```python
from build123d import *

# Parameters (mm, degrees)
SKETCH1_W            = 3.556
SKETCH1_H            = 2.794
SKETCH1_W_2          = 1.3716
SKETCH1_H_2          = 0.635
BOSS_EXTRUDE1_DEPTH  = 34.29
SKETCH2_R            = 9.525
BOSS_EXTRUDE2_DEPTH  = 8.255
SKETCH3_R            = 4.0005
BOSS_EXTRUDE3_DEPTH  = 13.081
SKETCH4_W            = 25.4
SKETCH4_H            = 16.9037
BOSS_EXTRUDE4_DEPTH  = 21.6662
SKETCH5_R            = 4.0005
BOSS_EXTRUDE5_DEPTH  = 13.081
SKETCH6_R            = 9.525
BOSS_EXTRUDE6_DEPTH  = 3.81
SKETCH7_W            = 19.177
SKETCH7_H            = 19.177
BOSS_EXTRUDE7_DEPTH  = 5.08
SKETCH8_R            = 3.175
BOSS_EXTRUDE8_DEPTH  = 15.494
SKETCH9_W            = 6.35
SKETCH9_H            = 6.35
BOSS_EXTRUDE9_DEPTH  = 6.35
SKETCH10_R           = 3.175
BOSS_EXTRUDE10_DEPTH = 3.175
BOSS_EXTRUDE11_DEPTH = 15.24
SKETCH12_R           = 3.175
BOSS_EXTRUDE12_DEPTH = 6.985
SKETCH13_W           = 15.9004
SKETCH13_H           = 15.875
BOSS_EXTRUDE13_DEPTH = 2.54
BOSS_EXTRUDE15_DEPTH = 2.54
CUT_EXTRUDE1_DEPTH   = 15
CUT_EXTRUDE2_DEPTH   = 15
FILLET1_R            = 1.27
SKETCH22_R           = 2.54
SKETCH22_R_2         = 0.127
CUT_EXTRUDE3_DEPTH   = 3.81
SKETCH22_3_R         = 0.127
CUT_EXTRUDE4_DEPTH   = 12.7
CUT_EXTRUDE7_DEPTH   = 5.08


with BuildPart() as part:
    # Sketch1 → Boss-Extrude1 (new body)
    with BuildSketch(Plane(origin=(0, 0, 0), x_dir=(1, 0, 0), z_dir=(0, 1, 0))):
        with Locations((1.778, -1.397)):
            Rectangle(SKETCH1_W, SKETCH1_H)
        with Locations((1.778, -1.397)):
            Rectangle(SKETCH1_W_2, SKETCH1_H_2, mode=Mode.SUBTRACT)
    extrude(amount=BOSS_EXTRUDE1_DEPTH)

    # Sketch2 → Boss-Extrude2 (add)
    with BuildSketch(Plane(origin=(0, 34.29, 0), x_dir=(1, 0, 0), z_dir=(0, 1, 0))):
        with Locations((1.778, -1.397)):
            Circle(SKETCH2_R)
    extrude(amount=BOSS_EXTRUDE2_DEPTH)

    # Sketch3 → Boss-Extrude3 (add)
    with BuildSketch(Plane(origin=(0, 42.545, 0), x_dir=(1, 0, 0), z_dir=(0, 1, 0))):
        with Locations((1.778, -1.397)):
            Circle(SKETCH3_R)
    extrude(amount=BOSS_EXTRUDE3_DEPTH)

    # Sketch4 → Boss-Extrude4 (add)
    with BuildSketch(Plane(origin=(0, 55.626, 0), x_dir=(1, 0, 0), z_dir=(0, 1, 0))):
        with Locations((1.778, -1.397)):
            Rectangle(SKETCH4_W, SKETCH4_H)
    extrude(amount=BOSS_EXTRUDE4_DEPTH)

    # Sketch5 → Boss-Extrude5 (add)
    with BuildSketch(Plane(origin=(0, 77.2922, 0), x_dir=(1, 0, 0), z_dir=(0, 1, 0))):
        with Locations((1.778, -1.397)):
            Circle(SKETCH5_R)
    extrude(amount=BOSS_EXTRUDE5_DEPTH)

    # Sketch6 → Boss-Extrude6 (add)
    with BuildSketch(Plane(origin=(0, 90.3732, 0), x_dir=(1, 0, 0), z_dir=(0, 1, 0))):
        with Locations((1.778, -1.397)):
            Circle(SKETCH6_R)
    extrude(amount=BOSS_EXTRUDE6_DEPTH)

    # Sketch7 → Boss-Extrude7 (add)
    with BuildSketch(Plane(origin=(0, 94.1832, 0), x_dir=(1, 0, 0), z_dir=(0, 1, 0))):
        with Locations((1.778, -1.397)):
            Rectangle(SKETCH7_W, SKETCH7_H)
    extrude(amount=BOSS_EXTRUDE7_DEPTH)

    # Sketch8 → Boss-Extrude8 (add)
    with BuildSketch(Plane(origin=(0, 99.2632, 0), x_dir=(1, 0, 0), z_dir=(0, 1, 0))):
        with Locations((1.778, 3.39725)):
            Circle(SKETCH8_R)
    extrude(amount=BOSS_EXTRUDE8_DEPTH)

    # Sketch9 → Boss-Extrude9 (add)
    with BuildSketch(Plane(origin=(0, 114.7572, 0), x_dir=(1, 0, 0), z_dir=(0, 1, 0))):
        with Locations((1.778, 3.39725)):
            Rectangle(SKETCH9_W, SKETCH9_H)
    extrude(amount=BOSS_EXTRUDE9_DEPTH)

    # Sketch10 → Boss-Extrude10 (add)
    with BuildSketch(Plane(origin=(0, 0, -6.57225), x_dir=(-1, 0, 0), z_dir=(0, 0, -1))):
        with Locations((-1.778, 117.9322)):
            Circle(SKETCH10_R)
    extrude(amount=BOSS_EXTRUDE10_DEPTH)

    # Sketch11 → Boss-Extrude11 (add)
    with BuildSketch(Plane(origin=(0, 0, -9.74725), x_dir=(-1, 0, 0), z_dir=(0, 0, -1))):
        Polygon((0.49502801, 113.9952), (2.76805602, 117.9322), (0.49502801, 121.8692), (-4.05102801, 121.8692), (-6.32405602, 117.9322), (-4.05102801, 113.9952), align=None)
    extrude(amount=BOSS_EXTRUDE11_DEPTH)

    # Sketch12 → Boss-Extrude12 (add)
    with BuildSketch(Plane(origin=(0, 0, -24.98725), x_dir=(-1, 0, 0), z_dir=(0, 0, -1))):
        with Locations((-1.778, 117.9322)):
            Circle(SKETCH12_R)
    extrude(amount=BOSS_EXTRUDE12_DEPTH)

    # Sketch13 → Boss-Extrude13 (add)
    with BuildSketch(Plane(origin=(0, 0, -7.05485), x_dir=(-1, 0, 0), z_dir=(0, 0, -1))):
        with Locations((-5.2578, 66.8147)):
            Rectangle(SKETCH13_W, SKETCH13_H)
    extrude(amount=BOSS_EXTRUDE13_DEPTH)

    # Sketch16 → Revolve1 (revolve)
    with BuildSketch(Plane(origin=(5.2578, 0, 0), x_dir=(0, 0, -1), z_dir=(1, 0, 0))):
        with BuildLine():
            Line((9.59485, 66.8147), (9.59485, 71.8947))
            Line((9.59485, 71.8947), (16.19885, 71.8947))
            Line((16.19885, 71.8947), (17.97685, 73.1647))
            Line((17.97685, 73.1647), (25.08885, 73.1647))
            Line((25.08885, 73.1647), (25.08885, 73.6727))
            Line((25.08885, 73.6727), (31.43885, 73.6727))
            ThreePointArc((31.43885, 73.6727), (33.469498821, 71.155053903), (34.48685, 68.0847))
            Line((34.48685, 68.0847), (34.74085, 68.0847))
            Line((34.74085, 68.0847), (34.74085, 66.8147))
            Line((34.74085, 66.8147), (9.59485, 66.8147))
        make_face()
    revolve(axis=Axis((5.2578, 66.8147, -9.59485), (0, 0, -1)))

    # Sketch17 → Boss-Extrude15 (add, symmetric)
    with BuildSketch(Plane(origin=(0, 107.0102, 0), x_dir=(1, 0, 0), z_dir=(0, 1, 0))):
        Polygon((6.470702988, 3.39725), (4.124351494, 7.46125), (-0.568351494, 7.46125), (-2.914702988, 3.39725), (-0.568351494, -0.66675), (4.124351494, -0.66675), align=None)
    extrude(amount=BOSS_EXTRUDE15_DEPTH, both=True)

    # Sketch20 → Cut-Extrude1 (cut)
    with BuildSketch(Plane.ZY):
        Polygon((0, 0), (0.762, 0), (0, 1.27), align=None)
        Polygon((2.794, 0), (2.794, 1.27), (2.032, 0), align=None)
    extrude(amount=-CUT_EXTRUDE1_DEPTH, mode=Mode.SUBTRACT)

    # Sketch21 → Cut-Extrude2 (cut)
    with BuildSketch(Plane(origin=(0, 0, 0), x_dir=(-1, 0, 0), z_dir=(0, 0, -1))):
        Polygon((-3.556, 1.27), (-3.556, 0), (-2.794, 0), align=None)
        Polygon((0, 1.27), (-0.762, 0), (0, 0), align=None)
    extrude(amount=-CUT_EXTRUDE2_DEPTH, mode=Mode.SUBTRACT)

    # Fillet1
    fillet1_edges = [part.edges().sort_by_distance(p)[0] for p in [
        (1.778, 34.29, 0),
        (0, 34.29, 1.397),
        (1.778, 34.29, 2.794),
        (3.556, 34.29, 1.397),
    ]]
    fillet(fillet1_edges, radius=FILLET1_R)

    # Sketch22 → Cut-Extrude3 (cut)
    with BuildSketch(Plane(origin=(0, 0, -31.97225), x_dir=(-1, 0, 0), z_dir=(0, 0, -1))):
        with Locations((-1.778, 117.9322)):
            Circle(SKETCH22_R)
        with Locations((-1.778, 117.9322)):
            Circle(SKETCH22_R_2, mode=Mode.SUBTRACT)
    extrude(amount=-CUT_EXTRUDE3_DEPTH, mode=Mode.SUBTRACT)

    # Sketch22_3 → Cut-Extrude4 (cut)
    with BuildSketch(Plane(origin=(0, 0, -31.97225), x_dir=(-1, 0, 0), z_dir=(0, 0, -1))):
        with Locations((-1.778, 117.9322)):
            Circle(SKETCH22_3_R)
    extrude(amount=-CUT_EXTRUDE4_DEPTH, mode=Mode.SUBTRACT)

    # Sketch25 → Cut-Extrude7 (cut)
    with BuildSketch(Plane.XY.offset(-17.78)):
        with BuildLine():
            Line((-0.49502801, 121.8692), (-1.63154216, 119.900699749))
            ThreePointArc((-1.63154216, 119.900699749), (-0.190500126, 121.341741942), (1.778, 121.8692))
            Line((1.778, 121.8692), (-0.49502801, 121.8692))
        make_face()
        with BuildLine():
            Line((4.05102801, 121.8692), (1.778, 121.8692))
            ThreePointArc((1.778, 121.8692), (3.746499994, 121.341742018), (5.187542007, 119.900700013))
            Line((5.187542007, 119.900700013), (4.05102801, 121.8692))
        make_face()
        with BuildLine():
            ThreePointArc((1.778, 113.9952), (-0.190500026, 114.522658), (-1.631542045, 115.963700052))
            Line((-1.631542045, 115.963700052), (-0.49502801, 113.9952))
            Line((-0.49502801, 113.9952), (1.778, 113.9952))
        make_face()
        with BuildLine():
            Line((-1.63154216, 119.900699749), (-2.76805602, 117.9322))
            Line((-2.76805602, 117.9322), (-1.631542045, 115.963700052))
            ThreePointArc((-1.631542045, 115.963700052), (-2.159, 117.932199885), (-1.63154216, 119.900699749))
        make_face()
        with BuildLine():
            ThreePointArc((5.18754197, 115.963699923), (3.746499961, 114.522657963), (1.778, 113.9952))
            Line((1.778, 113.9952), (4.05102801, 113.9952))
            Line((4.05102801, 113.9952), (5.18754197, 115.963699923))
        make_face()
        with BuildLine():
            ThreePointArc((5.715, 117.9322), (5.580849967, 116.913229376), (5.18754197, 115.963699923))
            Line((5.18754197, 115.963699923), (6.32405602, 117.9322))
            Line((6.32405602, 117.9322), (5.187542007, 119.900700013))
            ThreePointArc((5.187542007, 119.900700013), (5.580849976, 118.951170588), (5.715, 117.9322))
        make_face()
    extrude(amount=-CUT_EXTRUDE7_DEPTH, mode=Mode.SUBTRACT)


solid = part.part
```
Can you work these out from the model? Positions are in its coordinate system, mm. A direction names the side the tool comes from. Round coordinates to 2 decimals unless told otherwise and drop trailing zeros. Loops run counter-clockwise (first coordinate to the right, second up) from the corner with the lowest first, then second, coordinate; pieces in that order, holes last. Notation, with made-up numbers: M 25,48.25 L 48,48.25 A28 ccw 48,79.25 Z; hole C -0.75,29 d7. An arc over 180 degrees is marked long. Answer in a Markdown table with one row per item.
1. I'm going to push flat-ended pins straight in: pin 1 Ø4 at (x, y) = (1, 118) entering from -Z; pin 2 Ø6.5 at (x, y) = (-1.5, 68.5) entering from +Z; pin 3 Ø1.6 at (x, z) = (3, -2.5) entering from -Y. Where does each tip first touch, or does it pass through?
Established:
| item | result |
|---|---|
| pin 1 | z = -31.97 |
| pin 2 | z = 9.85 |
| pin 3 | y = 34.29 |
2. If we section it at B-B, the plane z = -12: Please give me the cut outline in (x, y), plus the area to 3 significant figures.
Established:
| item | result |
|---|---|
| outline | M -2.77,117.93 L -0.5,114 L 4.05,114 L 6.32,117.93 L 4.05,121.87 L -0.5,121.87 Z; C 5.26,66.81 d10.16 |
| area | 135 mm² |
3. If we section it at C-C, the plane x = -4.25: Please give me the cut outline in (y, z) (1 decimal).
Established:
| item | result |
|---|---|
| outline | M 34.3,-6 L 42.5,-6 L 42.5,8.8 L 34.3,8.8 Z; M 55.6,-7.1 L 77.3,-7.1 L 77.3,9.8 L 55.6,9.8 Z; M 90.4,-6 L 94.2,-6 L 94.2,-8.2 L 99.3,-8.2 L 99.3,11 L 94.2,11 L 94.2,8.8 L 90.4,8.8 Z |
4. If we section it at D-D, the plane y = 101: Please give me the cut outline in (x, z) (3 decimals).
Established:
| item | result |
|---|---|
| outline | C 1.778,-3.397 d6.35 |
5. If we section it at A-A, the plane y = 25.5: Please give me the cut outline in (x, z), plus the area to 3 significant figures.
Established:
| item | result |
|---|---|
| outline | M 0,0 L 3.56,0 L 3.56,2.79 L 0,2.79 Z; hole M 1.09,1.08 L 2.46,1.08 L 2.46,1.71 L 1.09,1.71 Z |
| area | 9.06 mm² |
6. On a 3-axis mill with a long thin cutter (end or side, diameter ignored), from which of +Z, -Z, +X, -X, +Y, -Y can I reach the whole of each face in a straight line? I mean faces 4 (the face through (4.953, 118, -3)), 5 (the face through (0, 120, -31.972)), 6 (the face through (2.466, 114.833, -28.431)). Say none if no direction works.
Established:
| item | result |
|---|---|
| face 4 | +Z, +X, +Y |
| face 5 | -Z, +X, -X, +Y |
| face 6 | -Z |
7. Please list where these lines run through material, in increasing order: line 1 (Y direction, x = 8.5, z = -1) (3 decimals); line 2 (Z direction, x = 1.5, y = 14); line 3 (Z direction, x = -7.5, y = 62.5). Write a range as from..to.
Established:
| item | result |
|---|---|
| line 1 | 34.29..42.545, 55.626..77.292, 90.373..99.263 |
| line 2 | 0..1.08, 1.71..2.79 |
| line 3 | -7.05..9.85 |
8. Thinking about a two-plate mould opening in Y: for faces 1 (the face through (-1, 77.292, -2)), 2 (the face through (2, 97, 10.986)), 3 (the face through (5.17, 119.93, -23.91)), which applies, pulls with the +Y half, pulls with the -Y half, needs draft (parallel to the pull), parting line crosses it, or undercut?
Established:
| item | result |
|---|---|
| face 1 | undercut |
| face 2 | needs draft |
| face 3 | pulls with the +Y half |
